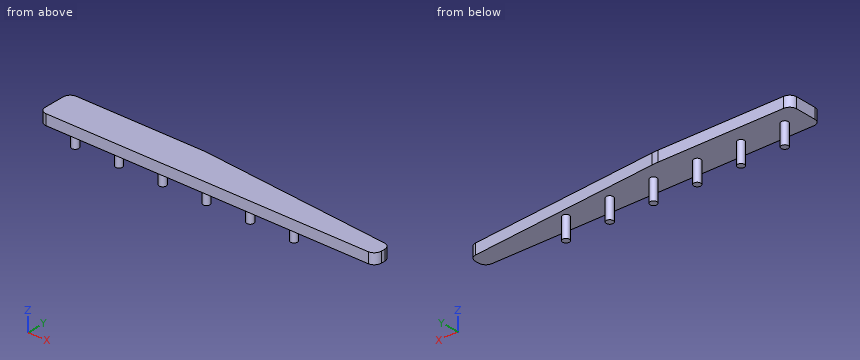
from build123d import *

# Parameters (mm, degrees)
BOSS_EXTRUDE1_DEPTH = 76.2
SKETCH2_R           = 25.4
BOSS_EXTRUDE2_DEPTH = 152.4
LPATTERN1_COUNT     = 6
LPATTERN1_PITCH     = 317.5


with BuildPart() as part:
    # Sketch1 → Boss-Extrude1 (new body)
    with BuildSketch(Plane.XY):
        with BuildLine():
            Line((-50.8, 0), (-2387.6, 0))
            ThreePointArc((-2387.6, 0), (-2423.521024484, 14.878975516), (-2438.4, 50.8))
            Line((-2438.4, 50.8), (-2438.4, 203.2))
            ThreePointArc((-2438.4, 203.2), (-2423.521024484, 239.121024484), (-2387.6, 254))
            Line((-2387.6, 254), (-1474.790405971, 254))
            ThreePointArc((-1474.790405971, 254), (-1452.64706645, 253.517164749), (-1430.545819782, 252.06957683))
            Line((-1430.545819782, 252.06957683), (-46.375541381, 131.054514896))
            ThreePointArc((-46.375541381, 131.054514896), (-13.34734657, 114.768669536), (0, 80.447557213))
            Line((0, 80.447557213), (0, 50.8))
            ThreePointArc((0, 50.8), (-14.878975516, 14.878975516), (-50.8, 0))
        make_face()
    extrude(amount=BOSS_EXTRUDE1_DEPTH)

    # Sketch2 → Boss-Extrude2 (add)
    with BuildSketch(Plane(origin=(0, 0, 0), x_dir=(-1, 0, 0), z_dir=(0, 0, -1))):
        with Locations(Location((2286, 127, 0), (0, 0, 180))):
            Circle(SKETCH2_R)
    boss_extrude2 = extrude(amount=BOSS_EXTRUDE2_DEPTH)

    # LPattern1: Boss-Extrude2 ×6
    with Locations(*[(i * LPATTERN1_PITCH, 0, 0) for i in range(1, LPATTERN1_COUNT)]):
        add(boss_extrude2)


solid = part.part
Design review of the part built by this model. Coordinates are the model's own, in mm. Coordinates: 2 decimals unless noted, no trailing zeros. Order: outer loops, then holes, each group sorted by start corner. A loop starts at its lowest first (then second) coordinate and runs counter-clockwise, first axis right, second up. Notation, with made-up numbers: M 58.5,89 L 87.5,89 A34 ccw 87.5,120 Z; hole C -8,81 d7. An arc over 180 degrees is marked long. Use a Markdown table: item, result.
(1) Add section A-A (z = -106). Give the boundary of the cut face in (x, y), then the cut area to 3 significant figures.
Worked answers:
| item | result |
|---|---|
| outline | C -2286,127 d50.8; C -1968.5,127 d50.8; C -1651,127 d50.8; C -1333.5,127 d50.8; C -1016,127 d50.8; C -698.5,127 d50.8 |
| area | 12,200 mm2 |
(2) Wall thickness on probe 1 along X at (y, z) = (115, -26); probe 2 along Z at (x, y) = (-1092, 81); probe 3 along Y at (x, z) = (-1163, 63): over which ranges is each line inside the solid? List them lowest first.
Worked answers:
| item | result |
|---|---|
| probe 1 | x = -2308.39 to -2263.61, -1990.89 to -1946.11, -1673.39 to -1628.61, -1355.89 to -1311.11, -1038.39 to -993.61, -720.89 to -676.11 |
| probe 2 | z = 0 to 76.2 |
| probe 3 | y = 0 to 228.68 |
(3) For P1, Ø1, axis at x = -1357, z = -82.5, coming from the -Y side; P2, Ø2, axis at x = -380, z = 6, coming from the +Y side; P3, Ø5, axis at y = 140, z = -109, coming from the +X side, all flat-tipped, find the tip position at first contact; note any pin that passes through.
Worked answers:
| item | result |
|---|---|
| P1 | stops at y = 116.22 |
| P2 | stops at y = 160.31 |
| P3 | stops at x = -675.37 |
(4) Add section D-D (x = -1586.5). Give the boundary of the cut face in (y, z).
Worked answers:
| item | result |
|---|---|
| outline | M 0,0 L 254,0 L 254,76.2 L 0,76.2 Z |
(5) Add section C-C (x = -1016). Give the boundary of the cut face in (y, z), then the cut area to 3 significant figures.
Worked answers:
| item | result |
|---|---|
| outline | M 0,0 L 101.6,0 L 101.6,-152.4 L 152.4,-152.4 L 152.4,0 L 215.83,0 L 215.83,76.2 L 0,76.2 Z |
| area | 24,200 mm2 |
(6) Add section B-B (x = -2286). Give the boundary of the cut face in (y, z).
Worked answers:
| item | result |
|---|---|
| outline | M 0,0 L 101.6,0 L 101.6,-152.4 L 152.4,-152.4 L 152.4,0 L 254,0 L 254,76.2 L 0,76.2 Z |
